Part model, mm, in its own coordinate system. A direction names the side the tool comes from. Give positions to 0.01 mm unless a question says otherwise; leave off trailing zeros. Write each loop counter-clockwise with the first axis right and the second up, starting at its lowest first coordinate (ties: lowest second). Pieces come first, ordered by that corner, then holes. Notation, with made-up numbers: M 0,17 L 39,17 A24 cw 39,32 Z; hole C 36,0.25 d11. An arc over 180 degrees is marked long. Use CSV: the item, a comma, the result in double quotes. Start each with the question number.
1. 3-axis set-ups, long thin cutter, end or side, ignore diameter. For faces 4 (the face through (14.4, 2.5, -22)), 5 (the face through (8, 1, -16.25)), 6 (the face through (18.55, 6.49, -18.52)): which of +Z, -Z, +X, -X, +Y, -Y reach the whole face in a straight line?
2. Drop flat-ended pins along their axis: pin 1 Ø1.3 at (x, y) = (21, 1) entering from -Z; pin 2 Ø0.6 at (y, z) = (1.5, -8) entering from -X; pin 3 Ø1.5 at (y, z) = (2.5, -26) entering from -X; pin 4 Ø0.9 at (x, y) = (7.5, 1.5) entering from +Z. Give the stop position or say it passes through.
3. Band-saw the part on A-A, the plane y = 0.5. Count the separate pieces of the cut face and the enclosed holes in it, then the cut area to 3 significant figures.
4. Mould opens along X. For faces 1 (the face through (24, 5, -14)), 2 (the face through (18.191, 0.986, -10.767)), 3 (the face through (29, 6, -14)) say: pulls with the +X half, pulls with the -X half, needs draft (parallel to the pull), parting line crosses it, or undercut.
5. Band-saw the part on C-C, the plane z = -10.5. List the corners of the cut face in (x, y), then the cut area to 3 significant figures.
6. Band-saw the part on D-D, the plane y = 2.5. List the corners of the cut face in (x, z).
7. Drill centre lines: line 1 along Z through (x, y) = (21.5, 1); line 2 along X through (y, z) = (6.5, -12.5); line 3 along Z through (x, y) = (11.25, 4.25). Where is each one in solid material? Low to high. Write a range as from..to.
8. Band-saw the part on B-B, the plane x = 15. List the corners of the cut face in (y, z), then the cut area to 3 significant figures.
from build123d import *

# Parameters (mm, degrees)
SKETCH1_W           = 29
SKETCH1_H           = 29
BOSS_EXTRUDE1_DEPTH = 7.5
SKETCH8_W           = 9
SKETCH8_H           = 9
CUT_EXTRUDE3_DEPTH  = 2
SKETCH9_W           = 29
SKETCH9_H           = 29
SKETCH9_W_2         = 15
SKETCH9_H_2         = 15
CUT_EXTRUDE4_DEPTH  = 5
CUT_EXTRUDE5_DEPTH  = 2
FILLET1_R           = 1.5875


with BuildPart() as part:
    # Sketch1 → Boss-Extrude1 (new body)
    with BuildSketch(Plane(origin=(0, 0, 0), x_dir=(1, 0, 0), z_dir=(0, 1, 0))):
        with Locations((14.5, 14.5)):
            Rectangle(SKETCH1_W, SKETCH1_H)
    extrude(amount=BOSS_EXTRUDE1_DEPTH)

    # Sketch8 → Cut-Extrude3 (cut)
    with BuildSketch(Plane(origin=(0, 7.5, 0), x_dir=(1, 0, 0), z_dir=(0, 1, 0))):
        with Locations((14.5, 14.5)):
            Rectangle(SKETCH8_W, SKETCH8_H)
    extrude(amount=-CUT_EXTRUDE3_DEPTH, mode=Mode.SUBTRACT)

    # Sketch9 → Cut-Extrude4 (cut)
    with BuildSketch(Plane.XZ):
        with Locations((14.5, -14.5)):
            Rectangle(SKETCH9_W, SKETCH9_H)
        with Locations((14.5, -14.5)):
            Rectangle(SKETCH9_W_2, SKETCH9_H_2, mode=Mode.SUBTRACT)
    extrude(amount=-CUT_EXTRUDE4_DEPTH, mode=Mode.SUBTRACT)

    # Sketch10 → Cut-Extrude5 (cut)
    with BuildSketch(Plane.XZ):
        Polygon((12.75, -7), (16.25, -7), (16.25, -8.825378798), (20.174621202, -12.75), (22, -12.75), (22, -16.25), (20.174621202, -16.25), (16.25, -20.174621202), (16.25, -22), (12.75, -22), (12.75, -20.174621202), (8.825378798, -16.25), (7, -16.25), (7, -12.75), (8.825378798, -12.75), (12.75, -8.825378798), align=None)
    extrude(amount=-CUT_EXTRUDE5_DEPTH, mode=Mode.SUBTRACT)

    # Fillet1
    fillet1_edges = [part.edges().sort_by_distance(p)[0] for p in [
        (10, 6.5, -10),
        (10, 6.5, -19),
        (19, 6.5, -19),
        (19, 6.5, -10),
        (12.75, 1, -8.825378798),
        (16.25, 1, -8.825378798),
        (20.174621202, 1, -12.75),
        (20.174621202, 1, -16.25),
        (16.25, 1, -20.174621202),
        (12.75, 1, -20.174621202),
        (8.825378798, 1, -16.25),
        (8.825378798, 1, -12.75),
        (0, 6.25, -29),
        (29, 6.25, -29),
        (29, 6.25, 0),
        (0, 6.25, 0),
    ]]
    fillet(fillet1_edges, radius=FILLET1_R)


solid = part.part
Output:
1,face 4,"-Z, +X, -X, -Y"
1,face 5,"+X, -X, -Y"
1,face 6,"+Y"
2,pin 1,"stops at z = -22"
2,pin 2,"stops at x = 7"
2,pin 3,"passes through"
2,pin 4,"stops at z = -7"
3,separate pieces,"4"
3,enclosed holes,"0"
3,area,"101 mm²"
4,face 1,"needs draft"
4,face 2,"undercut"
4,face 3,"pulls with the +X half"
5,outline,"M 0,5 L 7,5 L 7,0 L 11.08,0 L 11.08,2 L 17.92,2 L 17.92,0 L 22,0 L 22,5 L 29,5 L 29,7.5 L 18.57,7.5 L 18.57,5.5 L 10.43,5.5 L 10.43,7.5 L 0,7.5 Z"
5,area,"118 mm²"
6,outline,"M 7,-22 L 22,-22 L 22,-7 L 7,-7 Z"
7,line 1,"z = -22..-16.25, -12.75..-7"
7,line 2,"x = 0..10, 19..29"
7,line 3,"z = -22..-7"
8,outline,"M 2,-22 L 5,-22 L 5,-29 L 7.5,-29 L 7.5,-19 L 5.5,-19 L 5.5,-10 L 7.5,-10 L 7.5,0 L 5,0 L 5,-7 L 2,-7 Z"
8,area,"99.5 mm²"
